Work out the finished part from the listing and answer in its coordinate system (mm). A direction names the side the tool comes from. Coordinates: 2 decimals unless noted, no trailing zeros. Write each loop counter-clockwise with the first axis right and the second up, starting at its lowest first coordinate (ties: lowest second). Pieces come first, ordered by that corner, then holes. Notation, with made-up numbers: (-37, 33.5) - (-4, 33.5) arc R24 ccw to (-4, 43.5) - close; hole circle Ø11 at (21, 81.25). An arc over 180 degrees is marked (long way). Use one line per item in the form item = value. Start each with the question number.
Item 1: A cutting plane is placed at A-A (x = -19). Write down the section's boundary in (y, z) (3 decimals), then the cut area to 3 significant figures.
Item 2: Determine the mould class of faces 3 (the flat face through (-2, 13, 0)), 4 (the flat face through (-13, 25.476, 167)), 5 (the flat face through (-13, 3.175, 167)) for opening direction Y: released by +Y, released by -Y, zero draft, split by the parting line, or undercut.
Item 3: For faces 1 (the flat face through (-2, 13, 337.82)), 2 (the flat face through (-3.175, 13, 167)), determine the directions among +Z, -Z, +X, -X, +Y, -Y from which every point of the face is accessible in a straight line to the end or side of a thin tool.
Item 4: Given pin 1 (8 mm diameter, centred on y = 12.7, z = 12.7, fed in from -X), flat-ended and moving along its own axis, determine where the tip first touches the part or whether it passes through.
Item 5: Consider probe 1 along Y at (x, z) = (-0.55, 38.1); probe 2 along Y at (x, z) = (-19, 258) (3 decimals); probe 3 along X at (y, z) = (8.75, 253) (3 decimals). Determine where each line is inside the solid, lowest interval first.
from build123d import *

# Parameters (mm, degrees)
SKETCH1_W                    = 25.4
SKETCH1_H                    = 25.475595238
SKETCH1_W_2                  = 19.05
SKETCH1_H_2                  = 19.125595238
EXTRUDE_THIN1_DEPTH          = 337.82
F_10_0_1935_DIAMETER_HOLE1_D = 4.9149
F_10_0_1935_DIAMETER_HOLE2_D = 4.9149


with BuildPart() as part:
    # Sketch1 → Extrude-Thin1 (new body)
    with BuildSketch(Plane.XY):
        with Locations((-12.7, 12.737797619)):
            Rectangle(SKETCH1_W, SKETCH1_H)
        with Locations((-12.7, 12.737797619)):
            Rectangle(SKETCH1_W_2, SKETCH1_H_2, mode=Mode.SUBTRACT)
    extrude(amount=EXTRUDE_THIN1_DEPTH)

    # #10 (0.1935) Diameter Hole1 (through all)
    with Locations(Plane(origin=(0, 0, 0), x_dir=(-1, 0, 0), z_dir=(0, -1, 0))):
        with Locations((12.7, -25.4), (12.7, -12.7), (12.7, -38.1), (12.7, -299.72), (12.7, -312.42), (12.7, -325.12)):
            Hole(F_10_0_1935_DIAMETER_HOLE1_D / 2)

    # #10 (0.1935) Diameter Hole2 (through all)
    with Locations(Plane.ZY.offset(25.4)):
        with Locations((325.12, 12.666654514), (312.42, 12.666654514), (299.72, 12.666654514), (38.1, 12.7), (25.4, 12.7), (12.7, 12.7)):
            Hole(F_10_0_1935_DIAMETER_HOLE2_D / 2)


solid = part.part
Answer:
q1.outline = (0, 0) - (3.175, 0) - (3.175, 337.82) - (0, 337.82) - close; (22.301, 0) - (25.476, 0) - (25.476, 337.82) - (22.301, 337.82) - close
q1.area = 2,150 mm²
q2.face_3 = zero draft
q2.face_4 = released by +Y
q2.face_5 = undercut
q3.face_1 = +Z, +X, -X, +Y, -Y
q3.face_2 = +Z, -Z
q4.pin_1 = -25.4
q5.probe_1 = 0 to 10.24, 15.16 to 25.48
q5.probe_2 = 0 to 3.175, 22.301 to 25.476
q5.probe_3 = -25.4 to -22.225, -3.175 to 0
